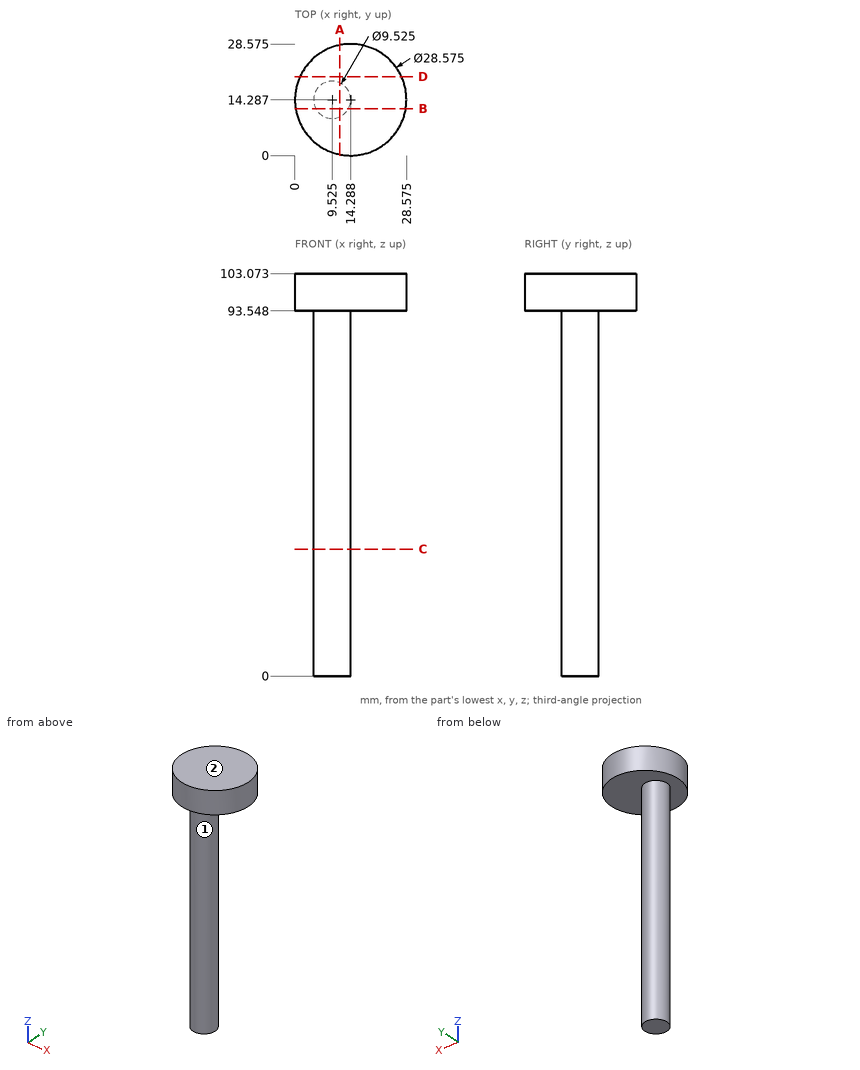
Geometry check sheet. Reference: drawing and pictorial views, mm from the part's lowest x, y, z. A direction names the side the tool comes from. Round coordinates to 2 decimals unless told otherwise and drop trailing zeros. Write each loop counter-clockwise with the first axis right and the second up, starting at its lowest first coordinate (ties: lowest second). Pieces come first, ordered by that corner, then holes.
1. Scan lines: L1, parallel to Z at x = 18, y = 6.5; L2, parallel to Y at x = 9.75, z = 15 (1 decimal); L3, parallel to Y at x = 13.25, z = 21 (1 decimal). Record each from-to range of solid material in increasing order.
2. Section check C-C on z = 32.5. Enter the section's corners in (x, y) (1 decimal).
3. Gauge pin test, flat ends, axial feed: P1, Ø8.5, axis at x = 20.5, y = 19, coming from the -Z side; P2, Ø2, axis at x = 10.5, z = 79.5, coming from the -Y side (1 decimal); P3, Ø2, axis at x = 12, z = 48, coming from the +Y side (1 decimal). Record the tip position at first contact, or that the pin passes through.
4. Section check B-B on y = 12. Enter the section's corners in (x, z) (1 decimal), plus the area to 3 significant figures.
5. Section check A-A on x = 11.5. Enter the section's corners in (y, z) (1 decimal), plus the area to 3 significant figures.
6. Section check D-D on y = 20.25. Enter the section's corners in (x, z).
7. Access from +Z, -Z, +X, -X, +Y, -Y to the whole of each face (thin tool, end or side, straight path). Record for the marked faces 1 and 2.
Answer:
1. L1: z = 93.55 to 103.07
1. L2: y = 9.5 to 19
1. L3: y = 11.3 to 17.3
2. outline: circle Ø9.5 at (9.5, 14.3)
3. P1: stops at z = 93.55
3. P2: stops at y = 9.5
3. P3: stops at y = 18.8
4. outline: (0.2, 93.5) - (5.3, 93.5) - (5.3, 0) - (13.7, 0) - (13.7, 93.5) - (28.4, 93.5) - (28.4, 103.1) - (0.2, 103.1) - close
4. area: 1,050 mm2
5. outline: (0.3, 93.5) - (10, 93.5) - (10, 0) - (18.6, 0) - (18.6, 93.5) - (28.3, 93.5) - (28.3, 103.1) - (0.3, 103.1) - close
5. area: 1,080 mm2
6. outline: (1.3, 93.55) - (27.27, 93.55) - (27.27, 103.07) - (1.3, 103.07) - close
7. face 1: -Z
7. face 2: +Z, +X, -X, +Y, -Y
